Part model, mm, in its own coordinate system. Face numbers are marked on the shaded views. A direction names the side the tool comes from. Coordinates: 2 decimals unless noted, no trailing zeros. Loops run counter-clockwise (first coordinate to the right, second up) from the corner with the lowest first, then second, coordinate; pieces in that order, holes last.
```python
from build123d import *

# Parameters (mm, degrees)
F0_W      = 50.8
F0_H      = 50.8
F1_DEPTH  = 7.62
F2_T      = -1.27
F3_W      = 16.2406819105
F3_H      = 1.27
F3_W_2    = 1.27
F3_H_2    = 5.9315557909
F3_W_3    = 24.0681569266
F3_W_4    = 1.640137285
F3_H_3    = 20.2985386211
F4_DEPTH  = 5.08
F5_W      = 7.2644
F5_H      = 1.27
F5_W_2    = 6.2484
F6_DEPTH  = 5.08
F7_R      = 1.27
F8_DEPTH  = 203.2
F9_W      = 11.2909469754
F9_H      = 1.27
F10_DEPTH = 5.08
F11_R     = 1.27
F12_DEPTH = 203.2


with BuildPart() as f1:
    # F0 (on Top) → F1 (new body)
    with BuildSketch(Plane.XY):
        with Locations((25.4, 25.4)):
            Rectangle(F0_W, F0_H)
    extrude(amount=F1_DEPTH)

    # F2
    f2_openings = [f1.faces().sort_by_distance(p)[0] for p in [
        (25.4, 25.4, 7.62),
    ]]
    offset(amount=F2_T, openings=f2_openings)

    # F3 (on face) → F4 (join)
    with BuildSketch(Plane.XY.offset(1.27)):
        Polygon((6.35, 39.3808744848), (6.35, 1.27), (7.62, 1.27), (7.62, 34.6140562403), (7.62, 35.8840562403), (7.62, 39.3808744848), align=None)
        with Locations((23.5678159714, 19.9215934223)):
            Rectangle(F3_W, F3_H)
        with Locations((17.7206453478, 11.2408155268)):
            Rectangle(F3_W_2, F3_H_2)
        Polygon((31.6881569266, 35.8840562403), (31.6881569266, 34.6140562403), (31.6881569266, 20.5565934223), (31.6881569266, 19.2865934223), (31.6881569266, 6.35), (32.9581569266, 6.35), (32.9581569266, 35.8840562403), align=None)
        with Locations((19.6540784633, 35.2490562403)):
            Rectangle(F3_W_3, F3_H)
        Polygon((38.0381569266, 21.5685386211), (42.9784730077, 21.5685386211), (44.6186102927, 21.5685386211), (44.6186102927, 22.8385386211), (38.0381569266, 22.8385386211), align=None)
        with Locations((43.7985416502, 11.4192693105)):
            Rectangle(F3_W_4, F3_H_3)
    extrude(amount=F4_DEPTH)

    # F5 (on Top) → F6 (join)
    with BuildSketch(Plane.XY):
        with Locations((40.4664789763, 42.1414506233)):
            Rectangle(F5_W, F5_H)
        with Locations((40.9744789763, 35.3089962697)):
            Rectangle(F5_W_2, F5_H)
    extrude(amount=F6_DEPTH)

    # F7 (on Top) → F8 (cut)
    with BuildSketch(Plane.XY):
        with Locations((3.81, 3.8211722858)):
            Circle(F7_R)
        with Locations((3.81, 8.3355149254)):
            Circle(F7_R)
        with Locations((3.81, 12.6183535904)):
            Circle(F7_R)
        with Locations((40.9753248096, 38.4839962697)):
            Circle(F7_R)
        with Locations((22.5706957281, 26.6243927181)):
            Circle(F7_R)
    extrude(amount=F8_DEPTH, mode=Mode.SUBTRACT)

    # F9 (on Top) → F10 (join)
    with BuildSketch(Plane.XY):
        with Locations((21.4138692245, 41.5160228109)):
            Rectangle(F9_W, F9_H)
    extrude(amount=F10_DEPTH)

    # F11 (on Top) → F12 (cut)
    with BuildSketch(Plane.XY):
        with Locations((24.7232858092, 10.317591019)):
            Circle(F11_R)
    extrude(amount=F12_DEPTH, mode=Mode.SUBTRACT)


solid = f1.part
```
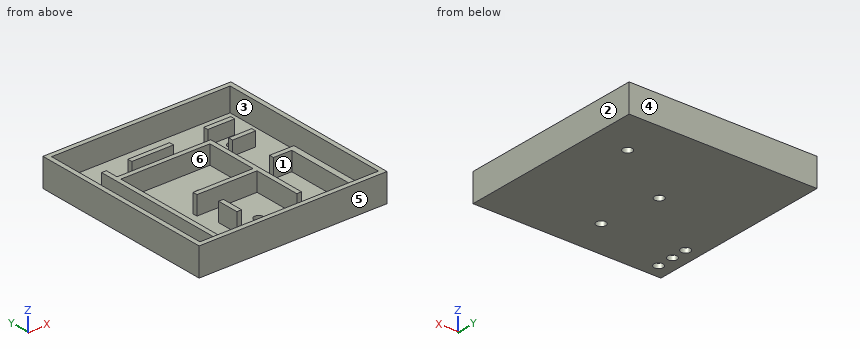
Q1. Tool access for the marked faces 5 and 6: list every direction of +Z, -Z, +X, -X, +Y, -Y with a clear straight run to the whole face (end or side of a thin tool).
Q2. Saw through at C-C (y = 44). List the corners of the cut face in (x, z), plus the area to 3 significant figures.
Q3. Saw through at A-A (z = 5.75). Count the separate pieces of the cut face and the enclosed holes in it, plus the area to 3 significant figures.
Q4. Mould opens along X. For the marked faces 1, 2, 3 and 4 say: released by +X, released by -X, zero draft, split by the parting line, or undercut.
Q5. Saw through at B-B (x = 3.81). List the corners of the cut face in (y, z).
Q6. Probe line 1 (X direction, y = 10.5, z = 5.5); line 2 (X direction, y = 36.5, z = 3.75); line 3 (Y direction, x = 22, z = 3.25). List the from-to ranges inside material, lowest first.
Q7. Drop flat-ended pins along their axis: P1, Ø1, axis at x = 17.5, y = 12, coming from the +Z side; P2, Ø3, axis at x = 23.5, z = 3, coming from the -Y side; P3, Ø3, axis at x = 25.5, y = 40, coming from the +Z side. Give the stop position or say it passes through.
Checked values:
1. face 5: +Z, -Z, +X, -X, -Y
1. face 6: +Z
2. outline: (0, 0) - (50.8, 0) - (50.8, 7.62) - (49.53, 7.62) - (49.53, 1.27) - (1.27, 1.27) - (1.27, 7.62) - (0, 7.62) - close
2. area: 80.6 mm2
3. separate pieces: 2
3. enclosed holes: 1
3. area: 438 mm2
4. face 1: undercut
4. face 2: released by +X
4. face 3: undercut
4. face 4: zero draft
5. outline: (0, 0) - (2.55, 0) - (2.55, 1.27) - (1.27, 1.27) - (1.27, 7.62) - (0, 7.62) - close; (5.09, 0) - (7.07, 0) - (7.07, 1.27) - (5.09, 1.27) - close; (9.61, 0) - (11.35, 0) - (11.35, 1.27) - (9.61, 1.27) - close; (13.89, 0) - (50.8, 0) - (50.8, 7.62) - (49.53, 7.62) - (49.53, 1.27) - (13.89, 1.27) - close
6. line 1: x = 0 to 1.27, 6.35 to 7.62, 17.09 to 18.36, 31.69 to 32.96, 42.98 to 44.62, 49.53 to 50.8
6. line 2: x = 0 to 1.27, 6.35 to 7.62, 49.53 to 50.8
6. line 3: y = 0 to 1.27, 19.29 to 20.56, 34.61 to 35.88, 40.88 to 42.15, 49.53 to 50.8
7. P1: stops at z = 6.35
7. P2: stops at y = 0
7. P3: stops at z = 5.08
